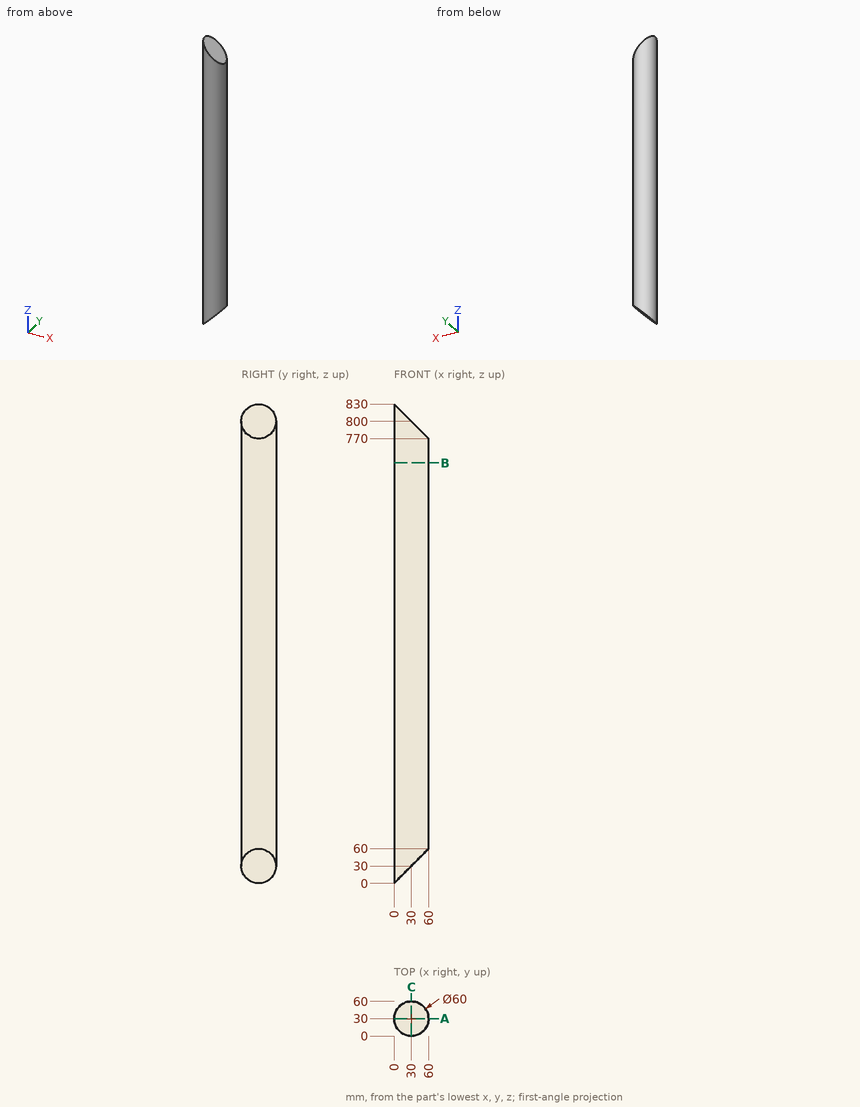
Check sheet for the drawn part. Datum: minimum x, y, z corner. Units: mm. Give positions to 0.01 mm unless a question says otherwise; leave off trailing zeros. Order: outer loops, then holes, each group sorted by start corner. A loop starts at its lowest first (then second) coordinate and runs counter-clockwise, first axis right, second up. Notation, with made-up numbers: (66, 49) - (104, 49) arc R14 ccw to (104, 64) - close; hole circle Ø10 at (77.25, 39). An arc over 180 degrees is marked (long way). Answer in a Markdown table with one row per item. Add a question column.
Q1. Cross-section at B-B, the plane z = 728. Enter the section's corners in (x, y).
Q2. Cross-section at A-A, the plane y = 30. Enter the section's corners in (x, z).
Q3. Cross-section at C-C, the plane x = 30. Enter the section's corners in (y, z).
Q4. Material ranges on probe 1 along Y at (x, z) = (31.5, 221.5); probe 2 along X at (y, z) = (32.5, 743.5); probe 3 along X at (y, z) = (22, 101.5), recorded low to high. Write a range as from..to.
Q5. Gauge pin test, flat ends, axial feed: pin 1 (8 mm diameter, centred on y = 43, z = 541, fed in from -X); pin 2 (12 mm diameter, centred on x = 50.5, y = 31, fed in from -Z); pin 3 (8 mm diameter, centred on y = 44, z = 654, fed in from +X); pin 4 (6 mm diameter, centred on y = 28, z = 686, fed in from +X). Record the tip position at first contact, or that the pin passes through.
Check values:
| question | item | result |
|---|---|---|
| 1 | outline | circle Ø60 at (30, 30) |
| 2 | outline | (0, 0) - (60, 60) - (60, 770) - (0, 830) - close |
| 3 | outline | (0, 30) - (60, 30) - (60, 800) - (0, 800) - close |
| 4 | probe 1 | y = 0.04..59.96 |
| 4 | probe 2 | x = 0.1..59.9 |
| 4 | probe 3 | x = 1.09..58.91 |
| 5 | pin 1 | stops at x = 1.38 |
| 5 | pin 2 | stops at z = 44.5 |
| 5 | pin 3 | stops at x = 58.28 |
| 5 | pin 4 | stops at x = 60 |
